The figure shows three views and two pictorial views of one solid part (mm, origin at its lowest corner). Answer the questions. A direction names the side the tool comes from. Coordinates: 2 decimals unless noted, no trailing zeros. Loops run counter-clockwise (first coordinate to the right, second up) from the corner with the lowest first, then second, coordinate; pieces in that order, holes last. Notation, with made-up numbers: M -13.5,84 L 39.5,84 A18 cw 39.5,106 Z; hole C 23,-28.75 d7. An arc over 180 degrees is marked long. Return JSON: item names as keys, results as strings. Group by question number.
1. The mould has two halves that part along X. Classify the marked faces 3, 4 and 5: pulls with the +X half, pulls with the -X half, needs draft (parallel to the pull), parting line crosses it, or undercut.
2. Section D-D (y = 4) is taken. Write down the section's boundary in (x, z), then the cut area to 3 significant figures.
3. Section C-C (z = 11) is taken. Write down the section's boundary in (x, y), then the cut area to 3 significant figures.
4. Given P1, Ø2, axis at x = 28.5, z = 5, coming from the +Y side; P2, Ø3, axis at y = 13, z = 3, coming from the +X side; P3, Ø4, axis at x = 12, z = 2, coming from the +Y side; P4, Ø10, axis at x = 17.5, y = 24, coming from the -Z side, each flat-ended and moving along its own axis, determine where each tip first touches the part or whether it passes through.
5. Straight lines are drawn through the part: L1, parallel to Y at x = 17, z = 5.5; L2, parallel to Z at x = 10, y = 3.5; L3, parallel to Y at x = 18, z = 5. For each, find the intervals that lie inside material, in ascending order. Write a range as from..to.
6. Section A-A (y = 17) is taken. Write down the section's boundary in (x, z).
7. Which of the six approach directions +Z, -Z, +X, -X, +Y, -Y give full straight-line access (tool end or side, diameter ignored) to the marked faces 1 and 2?
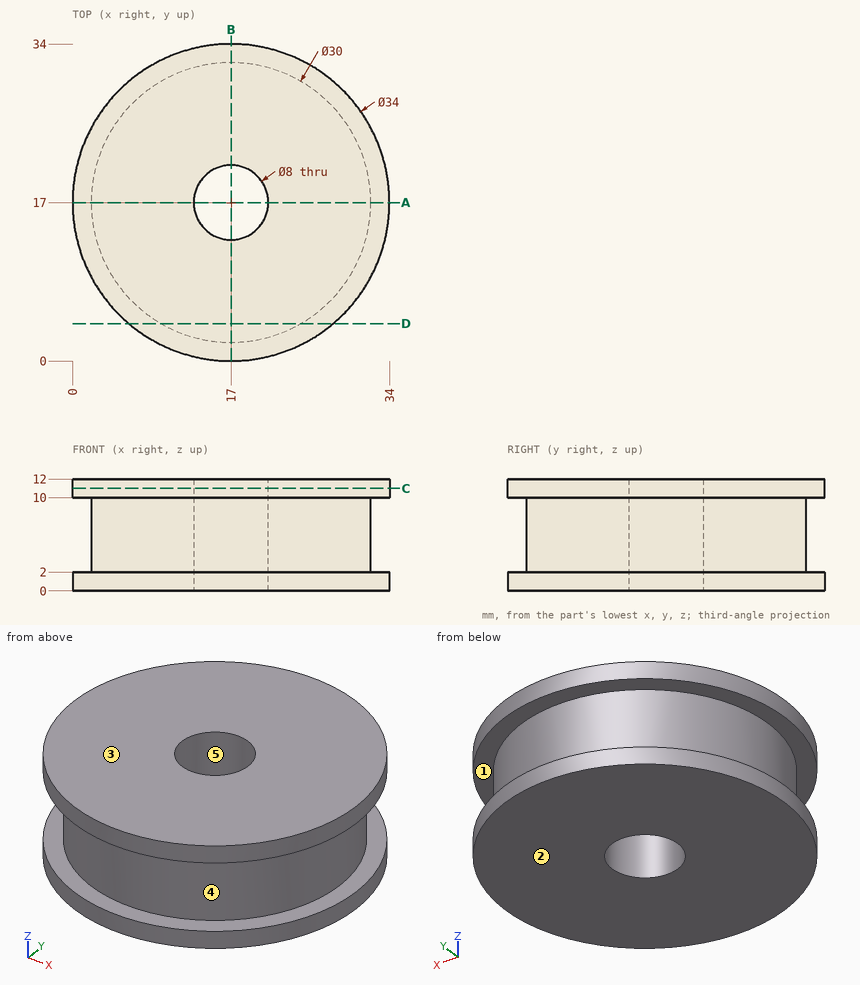
Worked out:
{
 "1": {"face 3": "needs draft", "face 4": "parting line crosses it", "face 5": "undercut"},
 "2": {"outline": "M 6.05,0 L 27.95,0 L 27.95,2 L 24.48,2 L 24.48,10 L 27.95,10 L 27.95,12 L 6.05,12 L 6.05,10 L 9.52,10 L 9.52,2 L 6.05,2 Z", "area": "207 mm^2"},
 "3": {"outline": "C 17,17 d34; hole C 17,17 d8", "area": "858 mm^2"},
 "4": {"P1": "y = 27.71", "P2": "x = 33.75", "P3": "y = 33.73", "P4": "z = 0"},
 "5": {"L1": "2..13, 21..32", "L2": "0..2, 10..12", "L3": "2.03..13.13, 20.87..31.97"},
 "6": {"outline": "M 0,0 L 13,0 L 13,12 L 0,12 L 0,10 L 2,10 L 2,2 L 0,2 Z; M 21,0 L 34,0 L 34,2 L 32,2 L 32,10 L 34,10 L 34,12 L 21,12 Z"},
 "7": {"face 1": "none", "face 2": "-Z, +X, -X, +Y, -Y"}
}
